```python
from build123d import *

# Parameters (mm, degrees)
SKETCH1_R           = 14.25
BOSS_EXTRUDE1_DEPTH = 0.5
SKETCH2_R           = 14.25
SKETCH2_R_2         = 13.75
BOSS_EXTRUDE2_DEPTH = 45
FILLET1_R           = 1
FILLET2_R           = 0.5


with BuildPart() as part:
    # Sketch1 → Boss-Extrude1 (new body)
    with BuildSketch(Plane(origin=(0, 0, 0), x_dir=(1, 0, 0), z_dir=(0, 1, 0))):
        with Locations(Location((0, 0, 0), (0, 0, 270))):
            Circle(SKETCH1_R)
    extrude(amount=BOSS_EXTRUDE1_DEPTH)

    # Sketch2 → Boss-Extrude2 (add)
    with BuildSketch(Plane(origin=(0, 0.5, 0), x_dir=(1, 0, 0), z_dir=(0, 1, 0))):
        with Locations(Location((0, 0, 0), (0, 0, 270))):
            Circle(SKETCH2_R)
        with Locations(Location((0, 0, 0), (0, 0, 90))):
            Circle(SKETCH2_R_2, mode=Mode.SUBTRACT)
    extrude(amount=BOSS_EXTRUDE2_DEPTH)

    # Fillet1
    fillet1_edges = [part.edges().sort_by_distance(p)[0] for p in [
        (0, 0, -14.25),
        (0, 0.5, 13.75),
    ]]
    fillet(fillet1_edges, radius=FILLET1_R)

    # Fillet2
    fillet2_edges = [part.edges().sort_by_distance(p)[0] for p in [
        (0, 45.5, -14.25),
    ]]
    fillet(fillet2_edges, radius=FILLET2_R - 0.0001)  # a hair under: the kernel refuses the full size


solid = part.part
```
Could you check a few things on this model? Use its own coordinates, in mm. Coordinates: 2 decimals unless noted, no trailing zeros. Write each loop counter-clockwise with the first axis right and the second up, starting at its lowest first coordinate (ties: lowest second). Pieces come first, ordered by that corner, then holes. Notation, with made-up numbers: (59, -14.5) -> (94, -14.5) arc R16 cw to (94, -2.5) -> close; hole circle Ø11 at (-31, 75). An arc over 180 degrees is marked (long way). Write item = value, one per line. Start each with the question number.
(1) I want a section at A-A (y = 17.5). Please give me the cut outline in (x, z).
(2) We'd pull the mould along X, two halves only. Please class faces 1 (the face through (-13.91, 22.69, -3.09)), 2 (the face through (0, 0, 0)), 3 (the face through (12.2, 23.19, -6.34)): released by +X, released by -X, zero draft, split by the parting line, or undercut.
(3) Will these pins go through, and if not, where does the flat tip stop? pin 1 (3 mm diameter, centred on x = -3.5, y = 30.5, fed in from -Z); pin 2 (4 mm diameter, centred on x = 10, y = 11.5, fed in from +Z); pin 3 (10 mm diameter, centred on x = -9.5, y = 6, fed in from -Z).
(4) I need wall thicknesses on line 1 (X direction, y = 14, z = 0); line 2 (Y direction, x = -11, z = -4); line 3 (X direction, y = 31, z = 9.75). Which ranges of each line are inside material? Lowest first, please. Write a range as [from, to].
Result set:
q1.outline = circle Ø28.5 at (0, 0); hole circle Ø27.5 at (0, 0)
q2.face_1 = split by the parting line
q2.face_2 = zero draft
q2.face_3 = undercut
q3.pin_1 = -14.11
q3.pin_2 = 11.79
q3.pin_3 = -13.52
q4.line_1 = [-14.25, -13.75], [13.75, 14.25]
q4.line_2 = [0, 0.5]
q4.line_3 = [-10.39, -9.7], [9.7, 10.39]
